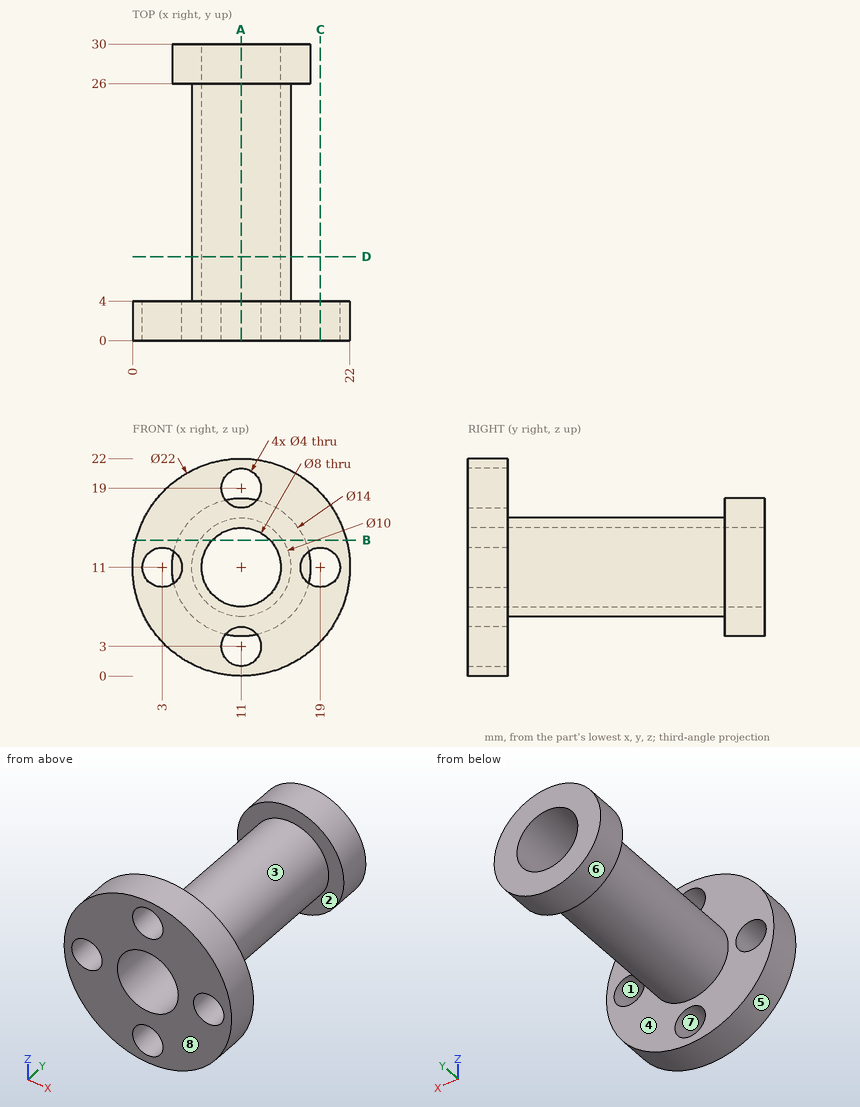
Geometry check sheet. Reference: drawing and pictorial views, mm from the part's lowest x, y, z. A direction names the side the tool comes from. Give positions to 0.01 mm unless a question says otherwise; leave off trailing zeros. Loops run counter-clockwise (first coordinate to the right, second up) from the corner with the lowest first, then second, coordinate; pieces in that order, holes last. Notation, with made-up numbers: (86, -3.5) -> (114, -3.5) arc R19 ccw to (114, 21.5) -> close; hole circle Ø7 at (17, 17.5). An arc over 180 degrees is marked (long way). Answer in a Markdown table with one row per item. Add a question column.
1) Gauge pin test, flat ends, axial feed: P1, Ø2, axis at x = 8, y = 13.5, coming from the -Z side; P2, Ø8, axis at x = 17, z = 7, coming from the -Y side; P3, Ø5, axis at y = 12, z = 17, coming from the -X side; P4, Ø3.5, axis at x = 19, z = 11, coming from the -Y side. Record the tip position at first contact, or that the pin passes through.
2) Cross-section at D-D on y = 8.5. Record the boundary of the cut face in (x, z), and give its area (3 significant figures).
3) Material ranges on probe 1 along Y at (x, z) = (14.5, 6); probe 2 along X at (y, z) = (1.7, 11); probe 3 along Z at (x, y) = (10.75, 23.25), recorded low to high. Write a range as from..to.
4) Cross-section at B-B on z = 13.75. Record the boundary of the cut face in (x, y).
5) Cross-section at C-C on x = 19. Record the boundary of the cut face in (y, z).
6) Cross-section at A-A on x = 11. Record the boundary of the cut face in (y, z).
7) Set-up check for the marked faces 4, 5, 6, 7 and 8: record each of +Z, -Z, +X, -X, +Y, -Y from which the full face is reachable in a straight line by a thin tool's end or side.
8) Draft check along Z on the marked faces 1, 2 and 3. Enter one of: pulls with the +Z half, pulls with the -Z half, needs draft (parallel to the pull), parting line crosses it, or undercut.
Outcome:
| question | item | result |
|---|---|---|
| 1 | P1 | stops at z = 6.42 |
| 1 | P2 | stops at y = 0 |
| 1 | P3 | stops at x = 7.43 |
| 1 | P4 | stops at y = 26 |
| 2 | outline | circle Ø10 at (11, 11); hole circle Ø8 at (11, 11) |
| 2 | area | 28.3 mm^2 |
| 3 | probe 1 | y = 0..4, 26..30 |
| 3 | probe 2 | x = 0..1, 5..7, 15..17, 21..22 |
| 3 | probe 3 | z = 6.01..7.01, 14.99..15.99 |
| 4 | outline | (0.35, 0) -> (8.1, 0) -> (8.1, 30) -> (4.56, 30) -> (4.56, 26) -> (6.82, 26) -> (6.82, 4) -> (0.35, 4) -> close; (13.9, 0) -> (21.65, 0) -> (21.65, 4) -> (15.18, 4) -> (15.18, 26) -> (17.44, 26) -> (17.44, 30) -> (13.9, 30) -> close |
| 5 | outline | (0, 3.45) -> (4, 3.45) -> (4, 9) -> (0, 9) -> close; (0, 13) -> (4, 13) -> (4, 18.55) -> (0, 18.55) -> close |
| 6 | outline | (0, 0) -> (4, 0) -> (4, 1) -> (0, 1) -> close; (0, 5) -> (4, 5) -> (4, 6) -> (26, 6) -> (26, 4) -> (30, 4) -> (30, 7) -> (0, 7) -> close; (0, 15) -> (30, 15) -> (30, 18) -> (26, 18) -> (26, 16) -> (4, 16) -> (4, 17) -> (0, 17) -> close; (0, 21) -> (4, 21) -> (4, 22) -> (0, 22) -> close |
| 7 | face 4 | none |
| 7 | face 5 | +Y, -Y |
| 7 | face 6 | +Y |
| 7 | face 7 | -Y |
| 7 | face 8 | +Z, -Z, +X, -X, -Y |
| 8 | face 1 | undercut |
| 8 | face 2 | needs draft |
| 8 | face 3 | parting line crosses it |
